Check sheet for the modelled part. Datum: model origin and axes. Units: mm. Face numbers are marked on the shaded views. Coordinates: 2 decimals unless noted, no trailing zeros. Loops run counter-clockwise (first coordinate to the right, second up) from the corner with the lowest first, then second, coordinate; pieces in that order, holes last.
```python
from build123d import *

# Parameters (mm, degrees)
SKETCH_1_W          = 44
SKETCH_1_H          = 42
EXTRUDE_1_DEPTH     = 9.5
SKETCH_2_R          = 11.5
CUT_EXTRUDE_1_DEPTH = 62.565006294
FILLET_1_R          = 3
SKETCH_5_R          = 1.5
CUT_EXTRUDE_2_DEPTH = 62.565006294


with BuildPart() as part:
    # 草图1 → 凸台-拉伸1 (new body)
    with BuildSketch(Plane(origin=(0, 0, 0), x_dir=(1, 0, 0), z_dir=(0, 1, 0))):
        with Locations((22, -21)):
            Rectangle(SKETCH_1_W, SKETCH_1_H)
    extrude(amount=EXTRUDE_1_DEPTH)

    # 草图2 → 切除-拉伸1 (cut, through all)
    with BuildSketch(Plane(origin=(0, 9.5, 0), x_dir=(1, 0, 0), z_dir=(0, 1, 0))):
        with Locations(Location((21.15, -20.85, 0), (0, 0, 270))):
            Circle(SKETCH_2_R)
    extrude(amount=-CUT_EXTRUDE_1_DEPTH, mode=Mode.SUBTRACT)

    # 圆角1
    fillet_1_edges = [part.edges().sort_by_distance(p)[0] for p in [
        (0, 4.75, 0),
        (44, 4.75, 0),
        (44, 4.75, 42),
        (0, 4.75, 42),
    ]]
    fillet(fillet_1_edges, radius=FILLET_1_R)

    # 草图5 → 切除-拉伸2 (cut, through all)
    with BuildSketch(Plane.XZ):
        with Locations(Location((36.65, 36.35, 0), (0, 0, 270))):
            Circle(SKETCH_5_R)
        with Locations(Location((5.65, 36.35, 0), (0, 0, 270))):
            Circle(SKETCH_5_R)
        with Locations(Location((5.65, 5.35, 0), (0, 0, 270))):
            Circle(SKETCH_5_R)
        with Locations(Location((36.65, 5.35, 0), (0, 0, 270))):
            Circle(SKETCH_5_R)
    extrude(amount=-CUT_EXTRUDE_2_DEPTH, mode=Mode.SUBTRACT)


solid = part.part
```
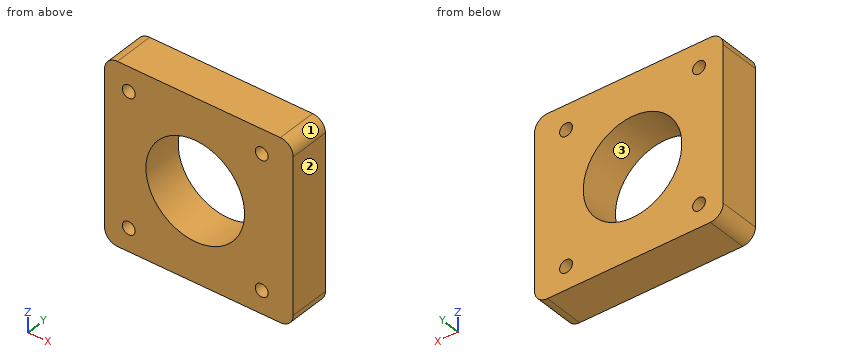
1) Depth check by flat-ended pin: pin 1 (3.5 mm diameter, centred on x = 36.65, z = 5.35, fed in from -Y). Enter the tip coordinate at first touch or a pass-through.
Answer sheet:
pin 1: stops at y = 0
2) Mould release check, pull along Z, two halves, no side actions. Record for the marked faces 1, 2 and 3: +Z half, -Z half, draft (parallel to the pull), parting line (faces both ways), or undercut.
Answer sheet:
face 1: +Z half
face 2: draft
face 3: undercut
3) Section check A-A on z = 36.35. Enter the section's corners in (x, y), plus the area to 3 significant figures.
Answer sheet:
outline: (0, 0) - (4.15, 0) - (4.15, 9.5) - (0, 9.5) - close; (7.15, 0) - (35.15, 0) - (35.15, 9.5) - (7.15, 9.5) - close; (38.15, 0) - (44, 0) - (44, 9.5) - (38.15, 9.5) - close
area: 361 mm2
4) Section check D-D on x = 36.65. Enter the section's corners in (y, z), plus the area to 3 significant figures.
Answer sheet:
outline: (0, 0) - (9.5, 0) - (9.5, 3.85) - (0, 3.85) - close; (0, 6.85) - (9.5, 6.85) - (9.5, 34.85) - (0, 34.85) - close; (0, 37.85) - (9.5, 37.85) - (9.5, 42) - (0, 42) - close
area: 342 mm2
5) Section check B-B on x = 21.15. Enter the section's corners in (y, z), plus the area to 4 significant figures.
Answer sheet:
outline: (0, 0) - (9.5, 0) - (9.5, 9.35) - (0, 9.35) - close; (0, 32.35) - (9.5, 32.35) - (9.5, 42) - (0, 42) - close
area: 180.5 mm2
6) Section check C-C on y = 1. Enter the section's corners in (x, z), plus the area to 3 significant figures.
Answer sheet:
outline: (0, 3) arc R3 ccw to (3, 0) - (41, 0) arc R3 ccw to (44, 3) - (44, 39) arc R3 ccw to (41, 42) - (3, 42) arc R3 ccw to (0, 39) - close; hole circle Ø3 at (5.65, 5.35); hole circle Ø3 at (5.65, 36.35); hole circle Ø23 at (21.15, 20.85); hole circle Ø3 at (36.65, 5.35); hole circle Ø3 at (36.65, 36.35)
area: 1,400 mm2
7) Scan lines: line 1 (X direction, y = 2.5, z = 36.35); line 2 (X direction, y = 1, z = 37); line 3 (X direction, y = 6.5, z = 20.85). Record each from-to range of solid material in increasing order.
Answer sheet:
line 1: x = 0 to 4.15, 7.15 to 35.15, 38.15 to 44
line 2: x = 0 to 4.3, 7 to 35.3, 38 to 44
line 3: x = 0 to 9.65, 32.65 to 44
